from build123d import *

# Parameters (mm, degrees)
SKETCH_W     = 31
SKETCH_H     = 10
SKETCH_R     = 1.625
PAD_DEPTH    = 1.6
SKETCH001_W  = 13.5
SKETCH001_H  = 5.75
PAD001_DEPTH = 12.4
SKETCH002_W  = 8.25
SKETCH002_H  = 2.56
POCKET_DEPTH = 14.001


with BuildPart() as part:
    # Sketch → Pad (new body)
    with BuildSketch(Plane.XY):
        Rectangle(SKETCH_W, SKETCH_H)
        with Locations((-12.675, 0)):
            Circle(SKETCH_R, mode=Mode.SUBTRACT)
        with Locations((12.675, 0)):
            Circle(SKETCH_R, mode=Mode.SUBTRACT)
    extrude(amount=PAD_DEPTH)

    # Sketch001 (on Face8 of Pad) → Pad001 (join)
    with BuildSketch(Plane.XY.offset(1.6)):
        Rectangle(SKETCH001_W, SKETCH001_H)
    extrude(amount=PAD001_DEPTH)

    # Sketch002 (on Face13 of Pad001) → Pocket (cut, through all)
    with BuildSketch(Plane.XY.offset(14)):
        Rectangle(SKETCH002_W, SKETCH002_H)
    extrude(amount=-POCKET_DEPTH, mode=Mode.SUBTRACT)


solid = part.part
The model under review builds one solid part; all positions refer to its coordinate system, in mm. A direction names the side the tool comes from. Round coordinates to 2 decimals unless told otherwise and drop trailing zeros. Loops run counter-clockwise (first coordinate to the right, second up) from the corner with the lowest first, then second, coordinate; pieces in that order, holes last. Notation, with made-up numbers: M 43.25,26 L 49.25,26 A9 cw 49.25,30 Z; hole C -9,86.5 d4. An arc over 180 degrees is marked long. Answer as CSV lines item,"result". Start each with the question number.
Item 1: For faces 4 (the face through (-15.5, 0, 1)), 5 (the face through (0, -2.875, 8)), 6 (the face through (-6.75, 0, 8)), 7 (the face through (0, 2.875, 8)), 8 (the face through (4.125, 0, 7)), list the 3-axis set-ups (+Z, -Z, +X, -X, +Y, -Y) from which the entire face can be reached by the end or side of a thin tool; tool diameter is ignored.
Item 2: Wall thickness on line 1 (Y direction, x = 0, z = 4.75) (3 decimals); line 2 (X direction, y = 1, z = 1.5) (3 decimals); line 3 (Z direction, x = -10.5, y = 0.75): over which ranges is each line inside the solid? List them lowest first. Write a range as [from, to].
Item 3: Consider section C-C (z = 1.25). Write out the cut boundary in (x, y) (3 decimals).
Item 4: Consider section D-D (z = 12.5). Write out the cut boundary in (x, y) (3 decimals), then the cut area to 3 significant figures.
Item 5: Mouldability with a two-part tool opening along X and no side actions: class faces 1 (the face through (6.75, 0, 8)), 2 (the face through (-11.125, 0.488, 0.789)), 3 (the face through (-0.2, 3.4, 1.6)) as released by +X, released by -X, zero draft, split by the parting line, or undercut.
Item 6: Consider section B-B (x = -2). Write out the cut boundary in (y, z) (3 decimals), then the cut area to 3 significant figures.
Item 7: Consider section A-A (y = 0). Write out the cut boundary in (x, z) (3 decimals), then the cut area to 3 significant figures.
Item 8: Insertion check: P1, Ø1.5, axis at y = 0, z = 8, coming from the +X side; P2, Ø2, axis at x = -8, z = 9, coming from the +Y side (1 decimal); P3, Ø4, axis at x = 12, y = 3, coming from the +Z side; P4, Ø2.5, axis at x = 1, z = 9.5, coming from the -Y side (3 decimals). Each pin has a flat end and moves straight along its axis. Give the tip position at first contact, or say it passes through.
Answer:
1,face 4,"+Z, -Z, -X, +Y, -Y"
1,face 5,"+Z, +X, -X, -Y"
1,face 6,"+Z, -X, +Y, -Y"
1,face 7,"+Z, +X, -X, +Y"
1,face 8,"+Z, -Z"
2,line 1,"y = [-2.875, -1.28], [1.28, 2.875]"
2,line 2,"x = [-15.5, -13.956], [-11.394, -4.125], [4.125, 11.394], [13.956, 15.5]"
2,line 3,"z = [0, 1.6]"
3,outline,"M -15.5,-5 L 15.5,-5 L 15.5,5 L -15.5,5 Z; hole C -12.675,0 d3.25; hole M -4.125,-1.28 L 4.125,-1.28 L 4.125,1.28 L -4.125,1.28 Z; hole C 12.675,0 d3.25"
4,outline,"M -6.75,-2.875 L 6.75,-2.875 L 6.75,2.875 L -6.75,2.875 Z; hole M -4.125,-1.28 L 4.125,-1.28 L 4.125,1.28 L -4.125,1.28 Z"
4,area,"56.5 mm^2"
5,face 1,"released by +X"
5,face 2,"undercut"
5,face 3,"zero draft"
6,outline,"M -5,0 L -1.28,0 L -1.28,14 L -2.875,14 L -2.875,1.6 L -5,1.6 Z; M 1.28,0 L 5,0 L 5,1.6 L 2.875,1.6 L 2.875,14 L 1.28,14 Z"
6,area,"51.5 mm^2"
7,outline,"M -15.5,0 L -14.3,0 L -14.3,1.6 L -15.5,1.6 Z; M -11.05,0 L -4.125,0 L -4.125,14 L -6.75,14 L -6.75,1.6 L -11.05,1.6 Z; M 4.125,0 L 11.05,0 L 11.05,1.6 L 6.75,1.6 L 6.75,14 L 4.125,14 Z; M 14.3,0 L 15.5,0 L 15.5,1.6 L 14.3,1.6 Z"
7,area,"91.1 mm^2"
8,P1,"stops at x = 6.75"
8,P2,"passes through"
8,P3,"stops at z = 1.6"
8,P4,"stops at y = -2.875"
